Part model, mm, in its own coordinate system. A direction names the side the tool comes from. Round coordinates to 2 decimals unless told otherwise and drop trailing zeros. Write each loop counter-clockwise with the first axis right and the second up, starting at its lowest first coordinate (ties: lowest second). Pieces come first, ordered by that corner, then holes.
1) Saw through at A-A on z = 6.5. Write the cut outline in (x, y).
2) Saw through at D-D on y = 27. Write the cut outline in (x, z).
3) Saw through at B-B on y = 7.5. Write the cut outline in (x, z).
4) Drill centre lines: L1, parallel to X at y = 7.5, z = 0.7; L2, parallel to X at y = 13, z = 0.75; L3, parallel to Y at x = 1.5, z = 4.75. Where is each one in solid material? Low to high.
5) Which spindle directions (+Z, -Z, +X, -X, +Y, -Y) get a long thin tool onto all of the face, cutting with end or side? Do faces 1 (the flat face through (26, 35.825, 8)), 2 (the flat face through (-10.65, 32, 1)), 3 (the flat face through (-20, 18, 8)), 4 (the cylindrical face through (-1.125, 35.606, 3.521)). Say none if no direction does.
6) Pull direction Y, two halves, no side cores. Call faces 5 (the cylindrical face through (-10.491, 5.538, 3.521)), 6 (the flat face through (25.245, 40.898, 2.465)), 7 (the flat face through (0, 24, 0)): +Y half, -Y half, draft (parallel to the pull), parting line (faces both ways), or undercut.
7) Flat gauge pins, fed straight in: pin 1 (3 mm diameter, centred on y = 24.5, z = 2, fed in from +X); pin 2 (2.5 mm diameter, centred on x = -26, z = 7, fed in from +Y); pin 3 (2 mm diameter, centred on y = 41, z = 4.5, fed in from -X). Where does each tip first touch, or does it go through?
8) Saw through at C-C on z = 3. Write the cut outline in (x, y), and give its area (3 significant figures).
```python
from build123d import *

# Parameters (mm, degrees)
SKETCH001_R     = 5.75
SKETCH001_R_2   = 3.5
SKETCH001_R_3   = 1.25
PAD_DEPTH       = 5
PAD001_DEPTH    = 8
PAD002_DEPTH    = 2
FILLET_R        = 1.5
POCKET_DEPTH    = 3
POCKET001_DEPTH = 3.5
FILLET001_R     = 2


with BuildPart() as part:
    # Sketch001 → Pad (new body)
    with BuildSketch(Plane.XY):
        with BuildLine():
            Line((-21.15, 47), (-28.65, 35.824688))
            Line((-28.65, 35.824688), (-20.173115, 2.999829))
            ThreePointArc((-20.173115, 2.999829), (-18.749596, 0.837668), (-16.300176, 0))
            Line((-16.300176, 0), (16.300176, 0))
            ThreePointArc((16.300176, 0), (18.749596, 0.837668), (20.173115, 2.999829))
            Line((20.173115, 2.999829), (28.65, 35.824688))
            Line((28.65, 35.824688), (21.15, 47))
            Line((21.15, 47), (-21.15, 47))
        make_face()
        with Locations((0, 17.53728)):
            Circle(SKETCH001_R, mode=Mode.SUBTRACT)
        with Locations((0, 41.412344)):
            Circle(SKETCH001_R_2, mode=Mode.SUBTRACT)
        with Locations((11, 41.412344)):
            Circle(SKETCH001_R_2, mode=Mode.SUBTRACT)
        with Locations((-8.941578, 7.5)):
            Circle(SKETCH001_R_3, mode=Mode.SUBTRACT)
        with Locations((-10.316813, 12.825292)):
            Circle(SKETCH001_R_3, mode=Mode.SUBTRACT)
        with Locations((-12.442175, 21.055288)):
            Circle(SKETCH001_R_3, mode=Mode.SUBTRACT)
        with Locations((-8.530434, 24.921588)):
            Circle(SKETCH001_R_3, mode=Mode.SUBTRACT)
        with Locations((8.941578, 7.5)):
            Circle(SKETCH001_R_3, mode=Mode.SUBTRACT)
        with Locations((10.316813, 12.825292)):
            Circle(SKETCH001_R_3, mode=Mode.SUBTRACT)
        with Locations((14.136115, 27.614693)):
            Circle(SKETCH001_R_3, mode=Mode.SUBTRACT)
        with Locations((15.511349, 32.939984)):
            Circle(SKETCH001_R_3, mode=Mode.SUBTRACT)
        with Locations((5.0822, 32.939984)):
            Circle(SKETCH001_R_3, mode=Mode.SUBTRACT)
        with Locations((-0.4178, 32.939984)):
            Circle(SKETCH001_R_3, mode=Mode.SUBTRACT)
        with BuildLine():
            ThreePointArc((-10.65, 33.324688), (-13.15, 35.824688), (-15.65, 33.324688))
            Line((-15.65, 33.324688), (-15.65, 30.324688))
            ThreePointArc((-15.65, 30.324688), (-13.15, 27.824688), (-10.65, 30.324688))
            Line((-10.65, 30.324688), (-10.65, 33.324688))
        make_face(mode=Mode.SUBTRACT)
    extrude(amount=PAD_DEPTH)

    # Sketch002 → Pad001 (join)
    with BuildSketch(Plane.XY):
        with BuildLine():
            Line((-25.551578, 35.824688), (-28.65, 35.824688))
            Line((-28.65, 35.824688), (-20.173115, 2.999829))
            ThreePointArc((-20.173115, 2.999829), (-18.749596, 0.837668), (-16.300176, 0))
            Line((-16.300176, 0), (-25.551578, 35.824688))
        make_face()
        with BuildLine():
            Line((28.65, 35.824688), (25.551578, 35.824688))
            Line((16.3, 0), (25.551578, 35.824688))
            ThreePointArc((16.3, 0), (18.749527, 0.837614), (20.173115, 2.999829))
            Line((28.65, 35.824688), (20.173115, 2.999829))
        make_face()
    extrude(amount=PAD001_DEPTH)

    # Sketch003 → Pad002 (join)
    with BuildSketch(Plane.XY.offset(8)):
        with BuildLine():
            Line((-16.300176, 0), (-12.168771, 0))
            Line((-12.168771, 0), (-21.420349, 35.824688))
            Line((-21.420349, 35.824688), (-28.65, 35.824688))
            Line((-28.65, 35.824688), (-20.173115, 2.999829))
            ThreePointArc((-20.173115, 2.999829), (-18.749596, 0.837668), (-16.300176, 0))
        make_face()
        with BuildLine():
            Line((16.300176, 0), (12.168771, 0))
            Line((12.168771, 0), (21.420349, 35.824688))
            Line((21.420349, 35.824688), (28.65, 35.824688))
            Line((28.65, 35.824688), (20.173115, 2.999829))
            ThreePointArc((16.300176, 0), (18.749596, 0.837668), (20.173115, 2.999829))
        make_face()
    extrude(amount=PAD002_DEPTH)

    # Fillet
    fillet_edges = [part.edges().sort_by_distance(p)[0] for p in [
        (-12.168771, 0, 9),
        (12.168771, 0, 9),
        (-21.420349, 35.824688, 9),
        (21.420349, 35.824688, 9),
    ]]
    fillet(fillet_edges, radius=FILLET_R)

    # Sketch004 (on DatumPlane) → Pocket (cut)
    with BuildSketch(Plane.XY.offset(5)):
        with BuildLine():
            Line((-11.362165, 6.874893), (-14.862762, 20.430181))
            ThreePointArc((-14.133267, 23.073669), (-14.85103, 21.849343), (-14.862762, 20.430181))
            Line((-14.133267, 23.073669), (-2.108891, 34.958365))
            ThreePointArc((0, 35.824688), (-1.139949, 35.599669), (-2.108891, 34.958365))
            Line((0, 35.824688), (14.319644, 35.824688))
            ThreePointArc((17.708466, 31.449539), (17.086685, 34.467931), (14.319644, 35.824688))
            Line((17.708466, 31.449539), (11.362165, 6.874893))
            ThreePointArc((8.941578, 5), (10.472466, 5.523543), (11.362165, 6.874893))
            Line((8.941578, 5), (-8.941578, 5))
            ThreePointArc((-11.362165, 6.874893), (-10.472466, 5.523543), (-8.941578, 5))
        make_face()
    extrude(amount=-POCKET_DEPTH, mode=Mode.SUBTRACT)

    # Sketch005 (on DatumPlane) → Pocket001 (cut)
    with BuildSketch(Plane.XY.offset(5)):
        with BuildLine():
            Line((-6.261651, 47), (-10.729413, 29.699582))
            ThreePointArc((-15.570587, 29.699582), (-13.15, 27.824688), (-10.729413, 29.699582))
            Line((-15.570587, 29.699582), (-20.038349, 47))
            Line((-20.038349, 47), (-6.261651, 47))
        make_face()
    extrude(amount=-POCKET001_DEPTH, mode=Mode.SUBTRACT)

    # Fillet001
    fillet001_edges = [part.edges().sort_by_distance(p)[0] for p in [
        (-21.15, 47, 2.5),
        (21.15, 47, 2.5),
    ]]
    fillet(fillet001_edges, radius=FILLET001_R)


solid = part.part
```
Completed:
1. outline: (-28.65, 35.82) - (-20.17, 3) arc R4 ccw to (-16.3, 0) - (-25.55, 35.82) - close; (16.3, 0) arc R4 ccw to (20.17, 3) - (28.65, 35.82) - (25.55, 35.82) - close
2. outline: (-26.37, 0) - (13.05, 0) - (13.05, 2) - (-10.16, 2) - (-10.16, 5) - (-23.27, 5) - (-23.27, 8) - (-19.14, 8) - (-19.14, 10) - (-26.37, 10) - close; (15.22, 0) - (26.37, 0) - (26.37, 10) - (19.14, 10) - (19.14, 8) - (23.27, 8) - (23.27, 5) - (16.56, 5) - (16.56, 2) - (15.22, 2) - close
3. outline: (-21.34, 0) - (-10.19, 0) - (-10.19, 2) - (-11.52, 2) - (-11.52, 5) - (-18.24, 5) - (-18.24, 8) - (-14.11, 8) - (-14.11, 10) - (-21.34, 10) - close; (-7.69, 0) - (7.69, 0) - (7.69, 2) - (-7.69, 2) - close; (10.19, 0) - (21.34, 0) - (21.34, 10) - (14.11, 10) - (14.11, 8) - (18.24, 8) - (18.24, 5) - (11.52, 5) - (11.52, 2) - (10.19, 2) - close
4. L1: x = -21.34 to -10.19, -7.69 to 7.69, 10.19 to 21.34
4. L2: x = -22.76 to -11.55, -9.08 to -3.53, 3.53 to 9.08, 11.55 to 22.76
4. L3: y = 0 to 5, 35.82 to 38.25, 44.57 to 47
5. face 1: +Z, +X, -X, +Y
5. face 2: +Z, -Z
5. face 3: +Y
5. face 4: +Z
6. face 5: undercut
6. face 6: +Y half
6. face 7: draft
7. pin 1: stops at x = 26.11
7. pin 2: stops at y = 35.82
7. pin 3: stops at x = -25.85
8. outline: (-28.65, 35.82) - (-20.17, 3) arc R4 ccw to (-16.3, 0) - (16.3, 0) arc R4 ccw to (20.17, 3) - (28.65, 35.82) - (21.74, 46.11) arc R2 ccw to (20.08, 47) - (-6.26, 47) - (-10.73, 29.7) arc R2.5 cw to (-15.57, 29.7) - (-20.04, 47) - (-20.08, 47) arc R2 ccw to (-21.74, 46.11) - close; hole (-14.86, 20.43) - (-11.36, 6.87) arc R2.5 ccw to (-8.94, 5) - (8.94, 5) arc R2.5 ccw to (11.36, 6.87) - (17.71, 31.45) arc R3.5 ccw to (14.32, 35.82) - (0, 35.82) arc R3 ccw to (-2.11, 34.96) - (-14.13, 23.07) arc R2.75 ccw to start; hole circle Ø7 at (0, 41.41); hole circle Ø7 at (11, 41.41)
8. area: 1,240 mm2
